from build123d import *

# Parameters (mm, degrees)
CIRPATTERN2_COUNT = 3
FILLET1_R         = 0.5


with BuildPart() as part:
    # Sketch1 → Revolve1 (revolve)
    with BuildSketch(Plane.XY):
        with BuildLine():
            Line((-27.2, 23.3), (-27.2, 22.25))
            Line((-27.2, 22.25), (-29, 22.25))
            Line((-29, 22.25), (-29, 22))
            Line((-29, 22), (-31, 22))
            Line((-31, 22), (-31, 15))
            Line((-31, 15), (-31.5, 15))
            Line((-31.5, 15), (-31.5, 11))
            Line((-31.5, 11), (-31.75, 11))
            Line((-31.75, 11), (-31.75, -14))
            Line((-31.75, -14), (-33.5, -14))
            Line((-33.5, -14), (-33.5, 21))
            ThreePointArc((-33.5, 21), (-32.621320344, 23.121320344), (-30.5, 24))
            Line((-30.5, 24), (-28.7, 24))
            Line((-28.7, 24), (-28.7, 23.3))
            Line((-28.7, 23.3), (-27.2, 23.3))
        make_face()
    revolve(axis=Axis((0, -0.222595104, 0), (0, -1, 0)))

    # Sketch4 → Cut-Revolve1 (revolve, cut)
    with BuildSketch(Plane.XY):
        Polygon((-33.5, -8), (-25.29746816, -8), (-25.29746816, -6.4), (-31.5, -6.4), (-33.5, -4.4), align=None)
    cut_revolve1 = revolve(axis=Axis((-29.768934642, -8, 0), (1, 0, 0)), mode=Mode.SUBTRACT)

    # CirPattern2: Cut-Revolve1 ×3 about axis
    cirpattern2_axis = Axis((0, 0, 0), (0, 1, 0))
    for i in range(1, CIRPATTERN2_COUNT):
        add(cut_revolve1.rotate(cirpattern2_axis, i * 360 / CIRPATTERN2_COUNT), mode=Mode.SUBTRACT)

    # Fillet1
    fillet1_edges = [part.edges().sort_by_distance(p)[0] for p in [
        (-33.324506796, -8, 3.424506796),
        (16.750000115, -11.6, 29.01185096),
        (16.749999851, -11.6, -29.011851113),
    ]]
    fillet(fillet1_edges, radius=FILLET1_R)


solid = part.part
Design review of the part built by this model. Coordinates are the model's own, in mm. A direction names the side the tool comes from. Round coordinates to 2 decimals unless told otherwise and drop trailing zeros. Write each loop counter-clockwise with the first axis right and the second up, starting at its lowest first coordinate (ties: lowest second). Pieces come first, ordered by that corner, then holes. Notation, with made-up numbers: (-39.5, -1.5) - (-34.5, -1.5) arc R18 cw to (-34.5, 27.5) - close; hole circle Ø3 at (-15.75, -26.75). An arc over 180 degrees is marked (long way). Use a Markdown table: item, result. Add a question column.
1. Wall thickness on probe 1 along Z at (x, y) = (0, 18.25); probe 2 along X at (y, z) = (9.5, 0.5): over which ranges is each line inside the solid? List them lowest first.
2. Clearance check with flat-ended pins moving along their axes: pin 1 (10 mm diameter, centred on x = 26.5, y = -5, fed in from -Z); pin 2 (2 mm diameter, centred on y = 5, z = 27, fed in from -X); pin 3 (12 mm diameter, centred on x = -23.5, y = -6, fed in from -Z). State where each tip first meets the part, or that it passes through.
3. We need section B-B (y = 6). State the section outline as (x, z) points, then the cut area to 3 significant figures.
4. For faces 1 (the face through (-11, 24, 27)), 2 (the face through (20.9, 15, 23.2)), 3 (the face through (-10.5, 23.3, 25.4)), list the 3-axis set-ups (+Z, -Z, +X, -X, +Y, -Y) from which the entire face can be reached by the end or side of a thin tool; tool diameter is ignored.
5. We need section C-C (y = -8). Count the separate pieces of the cut face and the enclosed holes in it, then the cut area to 3 significant figures.
Output:
| question | item | result |
|---|---|---|
| 1 | probe 1 | z = -33.5 to -31, 31 to 33.5 |
| 1 | probe 2 | x = -33.5 to -31.75, 31.75 to 33.5 |
| 2 | pin 1 | stops at z = -25.69 |
| 2 | pin 2 | stops at x = -21.12 |
| 2 | pin 3 | stops at z = -28.57 |
| 3 | outline | circle Ø67 at (0, 0); hole circle Ø63.5 at (0, 0) |
| 3 | area | 359 mm2 |
| 4 | face 1 | +Z, -Z, +X, -X, +Y |
| 4 | face 2 | -Y |
| 4 | face 3 | +Y |
| 5 | separate pieces | 3 |
| 5 | enclosed holes | 0 |
| 5 | area | 331 mm2 |
